```python
from build123d import *

# Parameters (mm, degrees)
SKETCH_1_R          = 12.5
SKETCH_1_R_2        = 6.25
EXTRUDE_1_DEPTH     = 3.5
SKETCH_2_R          = 1.55
CUT_EXTRUDE_1_DEPTH = 10
SKETCH_3_R          = 2.75
CUT_EXTRUDE_2_DEPTH = 3


with BuildPart() as part:
    # 草图1 → 凸台-拉伸1 (new body)
    with BuildSketch(Plane(origin=(0, 0, 0), x_dir=(1, 0, 0), z_dir=(0, 1, 0))):
        with Locations(Location((0, 0, 0), (0, 0, 270))):
            Circle(SKETCH_1_R)
        with Locations(Location((0, 0, 0), (0, 0, 270))):
            Circle(SKETCH_1_R_2, mode=Mode.SUBTRACT)
    extrude(amount=EXTRUDE_1_DEPTH)

    # 草图2 → 切除-拉伸1 (cut)
    with BuildSketch(Plane(origin=(0, 3.5, 0), x_dir=(1, 0, 0), z_dir=(0, 1, 0))):
        with Locations(Location((-10, 0, 0), (0, 0, 270))):
            Circle(SKETCH_2_R)
        with Locations(Location((0, 10, 0), (0, 0, 270))):
            Circle(SKETCH_2_R)
        with Locations(Location((10, 0, 0), (0, 0, 270))):
            Circle(SKETCH_2_R)
        with Locations(Location((0, -10, 0), (0, 0, 270))):
            Circle(SKETCH_2_R)
    extrude(amount=-CUT_EXTRUDE_1_DEPTH, mode=Mode.SUBTRACT)

    # 草图3 → 切除-拉伸2 (cut)
    with BuildSketch(Plane(origin=(0, 3.5, 0), x_dir=(1, 0, 0), z_dir=(0, 1, 0))):
        with Locations((-10, 0)):
            Circle(SKETCH_3_R)
        with Locations((0, 10)):
            Circle(SKETCH_3_R)
        with Locations((10, 0)):
            Circle(SKETCH_3_R)
        with Locations((0, -10)):
            Circle(SKETCH_3_R)
    extrude(amount=-CUT_EXTRUDE_2_DEPTH, mode=Mode.SUBTRACT)


solid = part.part
```
Input: part model. Units: mm. Frame: model coordinates. A direction names the side the tool comes from. Round coordinates to 2 decimals unless told otherwise and drop trailing zeros. Loops run counter-clockwise (first coordinate to the right, second up) from the corner with the lowest first, then second, coordinate; pieces in that order, holes last. Notation, with made-up numbers: (23, 43.25) -> (70, 43.25) arc R28 ccw to (70, 66.25) -> close; hole circle Ø6 at (43, -7). An arc over 180 degrees is marked (long way). One line per item, written item: value.
(1) Section A-A (z = -10). Return the cut outline in (x, y), plus the area to 4 significant figures.
Geometry check:
outline: (-7.5, 0) -> (-1.55, 0) -> (-1.55, 0.5) -> (-2.75, 0.5) -> (-2.75, 3.5) -> (-7.5, 3.5) -> close; (1.55, 0) -> (7.5, 0) -> (7.5, 3.5) -> (2.75, 3.5) -> (2.75, 0.5) -> (1.55, 0.5) -> close
area: 34.45 mm2
(2) Material intervals for line 1 (X direction, y = 0.25, z = 0); line 2 (Z direction, x = -10, y = 2.5); line 3 (Z direction, x = 0.5, y = 2.9), sorted ascending. Write a range as [from, to].
Geometry check:
line 1: [-12.5, -11.55], [-8.45, -6.25], [6.25, 8.45], [11.55, 12.5]
line 2: [-7.5, -2.75], [2.75, 7.5]
line 3: [-7.3, -6.23], [6.23, 7.3]
(3) Section C-C (x = -9.25). Return the cut outline in (y, z), plus the area to 3 significant figures.
Geometry check:
outline: (0, -8.41) -> (3.5, -8.41) -> (3.5, -2.65) -> (0.5, -2.65) -> (0.5, -1.36) -> (0, -1.36) -> close; (0, 1.36) -> (0.5, 1.36) -> (0.5, 2.65) -> (3.5, 2.65) -> (3.5, 8.41) -> (0, 8.41) -> close
area: 41.6 mm2
(4) Mould query, pull axis Z, two halves, no side actions, for faces 3 (the face through (6, 3.5, -3)), 4 (the face through (3.755, 1.726, 11.923)), 5 (the face through (-11.513, 0.253, -0.336)). Classes: pulls with the +Z half, pulls with the -Z half, needs draft (parallel to the pull), parting line crosses it, or undercut.
Geometry check:
face 3: needs draft
face 4: parting line crosses it
face 5: undercut
(5) Section B-B (z = 0). Return the cut outline in (x, y), plus the area to 3 significant figures.
Geometry check:
outline: (-12.5, 0) -> (-11.55, 0) -> (-11.55, 0.5) -> (-12.5, 0.5) -> close; (-8.45, 0) -> (-6.25, 0) -> (-6.25, 3.5) -> (-7.25, 3.5) -> (-7.25, 0.5) -> (-8.45, 0.5) -> close; (6.25, 0) -> (8.45, 0) -> (8.45, 0.5) -> (7.25, 0.5) -> (7.25, 3.5) -> (6.25, 3.5) -> close; (11.55, 0) -> (12.5, 0) -> (12.5, 0.5) -> (11.55, 0.5) -> close
area: 9.15 mm2
(6) Section D-D (x = 0). Return the cut outline in (y, z), plus the area to 3 significant figures.
Geometry check:
outline: (0, -12.5) -> (0.5, -12.5) -> (0.5, -11.55) -> (0, -11.55) -> close; (0, -8.45) -> (0.5, -8.45) -> (0.5, -7.25) -> (3.5, -7.25) -> (3.5, -6.25) -> (0, -6.25) -> close; (0, 6.25) -> (3.5, 6.25) -> (3.5, 7.25) -> (0.5, 7.25) -> (0.5, 8.45) -> (0, 8.45) -> close; (0, 11.55) -> (0.5, 11.55) -> (0.5, 12.5) -> (0, 12.5) -> close
area: 9.15 mm2
(7) Pin query (flat end, axial travel): pin 1 (2 mm diameter, centred on y = 1.5, z = 8, fed in from -X); pin 2 (3.5 mm diameter, centred on x = 10, z = 0, fed in from +Y); pin 3 (1 mm diameter, centred on x = -9.5, y = 0.5, fed in from +Z). Return the tip coordinate at first contact, or that it passes through.
Geometry check:
pin 1: x = -10.36
pin 2: y = 0.5
pin 3: z = 8.67
(8) Set-up query: faces 1 (the face through (1.88, 1.73, 5.96)), 2 (the face through (1.2, 0.5, -8.7)). Return all of +Z, -Z, +X, -X, +Y, -Y with unobstructed straight access to the full face (end or side cutting, diameter ignored); none if empty.
Geometry check:
face 1: +Y, -Y
face 2: +Y
